The model under review builds one solid part; all positions refer to its coordinate system, in mm. Face numbers are marked on the shaded views. A direction names the side the tool comes from. Give positions to 0.01 mm unless a question says otherwise; leave off trailing zeros. Loops run counter-clockwise (first coordinate to the right, second up) from the corner with the lowest first, then second, coordinate; pieces in that order, holes last. Notation, with made-up numbers: M -34.75,52.25 L -14.75,52.25 A13 cw -14.75,72.25 Z; hole C 26,36 d2. An arc over 180 degrees is marked long. Write item = value, one per line. Start each with the question number.
1. We need section D-D on y = 7.5. Give the boundary of the cut face in (x, z).
2. For pin 1 (3 mm diameter, centred on y = -20, z = 2.5, fed in from +X); pin 2 (1.2 mm diameter, centred on y = 20, z = 2.5, fed in from -X); pin 3 (0.7 mm diameter, centred on y = -19.5, z = 3, fed in from +X), all flat-tipped, find the tip position at first contact; note any pin that passes through.
3. We need section A-A on x = 9.5. Give the boundary of the cut face in (y, z).
4. Draft analysis for pull direction X (two halves, no side actions). For the marked faces 3 and 4, state which applies: pulls with the +X half, pulls with the -X half, needs draft (parallel to the pull), parting line crosses it, or undercut.
5. For the marked faces 1 and 2, list the 3-axis set-ups (+Z, -Z, +X, -X, +Y, -Y) from which the entire face can be reached by the end or side of a thin tool; tool diameter is ignored.
6. Wall thickness on line 1 along Y through (x, z) = (27.9, 2.5); line 2 along Y through (x, z) = (11, 4.45); line 3 along Z through (x, y) = (27, 20): over which ranges is each line inside the solid? List them lowest first. Write a range as from..to.
7. We need section C-C on z = 2.5. Count the separate pieces of the cut face and the enclosed holes in it, then the cut area to 3 significant figures.
8. We need section B-B on y = 0. Give the boundary of the cut face in (x, z), then the cut area to 3 significant figures.
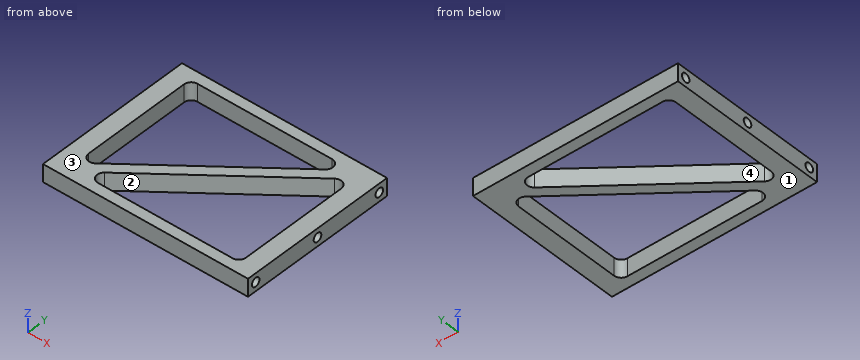
Autodesk Inventor part; units mm, degrees
ref_plane "YZ Plane" through (0, 0, 0) normal (1, 0, 0) x (0, 1, 0)
ref_plane "XZ Plane" through (0, 0, 0) normal (0, 1, 0) x (-1, 0, 0)
ref_plane "XY Plane" through (0, 0, 0) normal (0, 0, 1) x (1, 0, 0)
sketch "スケッチ1" plane through (0, 0, 0) normal (0, 0, 1) x (1, 0, 0)
  line L0 (-29.15, 22.5) -> (29.15, 22.5)
  line L1 (29.15, 22.5) -> (29.15, -22.5)
  line L2 (29.15, -22.5) -> (-29.15, -22.5)
  line L3 (-29.15, -22.5) -> (-29.15, 22.5)
  line L4 (-24.15, 19.5) -> (24.15, 19.5) construction
  line L5 (24.15, 19.5) -> (24.15, -19.5) construction
  line L6 (24.15, -19.5) -> (-24.15, -19.5) construction
  line L7 (-24.15, -19.5) -> (-24.15, 19.5) construction
  line L8 (24.15, 19.5) -> (-24.15, -19.5) construction
  line L9 (-24.15, -17.5721) -> (-24.15, 19.5)
  line L10 (-24.15, 19.5) -> (21.7623, 19.5)
  line L11 (21.7623, 19.5) -> (-24.15, -17.5721)
  line L12 (-21.7623, -19.5) -> (24.15, -19.5)
  line L13 (24.15, -19.5) -> (24.15, 17.5721)
  line L14 (24.15, 17.5721) -> (-21.7623, -19.5)
  line L15 (-29.15, 20) -> (29.15, 20) construction
  line L16 (29.15, -20) -> (-29.15, -20) construction
  line L17 (29.15, 20) -> (29.15, -20) construction
  point P0 (0, 0)
  point P1 (0, 19.5)
  point P2 (0, 22.5)
  point P3 (24.15, 0)
  point P4 (29.15, 0)
  dimension "d0" = 5
  dimension "d1" = 3
  dimension "d2" = 1.5
  dimension "d3" = 40
  dimension "d4" = 2.5
  dimension "d19" = 58.3
extrude "押し出し1" add sketch "スケッチ1" along normal blind 5
sketch "スケッチ2" plane through (29.15, -22.5, 0) normal (1, 0, 0) x (0, 0, -1)
  line L0 (0, 45) -> (-5, 45)
  line L1 (-5, 0) -> (-5, 45)
  line L2 (0, 22.5) -> (-5, 22.5) construction
  point P0 (-2.5, 2.5)
  point P1 (-2.5, 22.5)
  point P2 (-2.5, 42.5)
  point P3 (-2.5, 45)
  dimension "d7" = 40
hole "穴1" at (29.15, -20, 2.5) at (29.15, 0, 2.5) at (29.15, 20, 2.5) direction (-1, 0, 0) diameter 2.459 depth 3
mirror "ミラー1" about plane through (0, 0, 0) normal (1, 0, 0) of "穴1"
fillet "フィレット1" radius 2 6 edges at (-21.7623, -19.5, 2.5) (-24.15, -17.5721, 2.5) (24.15, 17.5721, 2.5) (24.15, -19.5, 2.5) (-24.15, 19.5, 2.5) (21.7623, 19.5, 2.5)
equation "\"d3\" = d11_1"
properties part number "リンク_ふくらはぎ_サブフレーム_1_1(予備案)" material "アルミニウム 2014-T4"
Final values:
q1.outline = M -29.15,0 L -24.15,0 L -24.15,5 L -29.15,5 Z; M 6.9,0 L 11.68,0 L 11.68,5 L 6.9,5 Z; M 24.15,0 L 29.15,0 L 29.15,5 L 24.15,5 Z
q2.pin_1 = 29.15
q2.pin_2 = -26.15
q2.pin_3 = 26.15
q3.outline = M -22.5,0 L -19.5,0 L -19.5,5 L -22.5,5 Z; M 5.74,0 L 9.6,0 L 9.6,5 L 5.74,5 Z; M 19.5,0 L 22.5,0 L 22.5,5 L 19.5,5 Z
q4.face_3 = needs draft
q4.face_4 = undercut
q5.face_1 = -Z, +X, -X, +Y, -Y
q5.face_2 = +Z, -Z
q6.line_1 = -22.5..-21.23, -18.77..-1.23, 1.23..18.77, 21.23..22.5
q6.line_2 = -22.5..-19.5, 6.95..10.81, 19.5..22.5
q6.line_3 = 0..1.27, 3.73..5
q7.separate_pieces = 1
q7.enclosed_holes = 2
q7.area = 899 mm²
q8.outline = M -29.15,0 L -24.15,0 L -24.15,5 L -29.15,5 L -29.15,3.73 L -26.15,3.73 L -26.15,1.27 L -29.15,1.27 Z; M -2.39,0 L 2.39,0 L 2.39,5 L -2.39,5 Z; M 24.15,0 L 29.15,0 L 29.15,1.27 L 26.15,1.27 L 26.15,3.73 L 29.15,3.73 L 29.15,5 L 24.15,5 Z
q8.area = 59.1 mm²
